Autodesk Inventor part; units mm, degrees
ref_plane "YZ Plane" through (0, 0, 0) normal (1, 0, 0) x (0, 1, 0)
ref_plane "XZ Plane" through (0, 0, 0) normal (0, 1, 0) x (-1, 0, 0)
ref_plane "XY Plane" through (0, 0, 0) normal (0, 0, 1) x (1, 0, 0)
sketch "Sketch1" plane through (0, 0, 0) normal (0, 1, 0) x (-1, 0, 0)
  line L0 (0, 0) -> (-36, 0)
  line L1 (-36, 0) -> (-36, -36)
  line L2 (-36, -36) -> (0, -36)
  line L3 (0, -36) -> (0, 0)
  circle A0 centre (-1.9445, -34.0555) radius 1.5
  circle A1 centre (-34.0555, -34.0555) radius 1.5
  circle A2 centre (-1.9445, -1.9445) radius 1.5
  circle A3 centre (-34.0555, -1.9445) radius 1.5
  line L4 (-6.1012, -34.6884) -> (-8.9666, -34.6884)
  line L5 (-8.9666, -34.6884) -> (-8.9666, -32.1278)
  line L6 (-8.9666, -32.1278) -> (-6.1012, -32.1278)
  line L7 (-6.1012, -32.1278) -> (-6.1012, -34.6884)
  line L8 (-11.5272, -34.6884) -> (-14.4536, -34.6884)
  line L9 (-14.4536, -34.6884) -> (-14.4536, -32.1278)
  line L10 (-14.4536, -32.1278) -> (-11.5272, -32.1278)
  line L11 (-11.5272, -32.1278) -> (-11.5272, -34.6884)
  line L12 (-17.5019, -34.6884) -> (-20.6111, -34.6884)
  line L13 (-20.6111, -34.6884) -> (-20.6111, -32.1278)
  line L14 (-20.6111, -32.1278) -> (-17.5019, -32.1278)
  line L15 (-17.5019, -32.1278) -> (-17.5019, -34.6884)
  line L16 (-23.9642, -34.6884) -> (-27.6831, -34.6884)
  line L17 (-27.6831, -34.6884) -> (-27.6831, -32.1278)
  line L18 (-27.6831, -32.1278) -> (-23.9642, -32.1278)
  line L19 (-23.9642, -32.1278) -> (-23.9642, -34.6884)
  line L20 (-34.6332, -30.055) -> (-31.9508, -30.055)
  line L21 (-31.9508, -30.055) -> (-31.9508, -27.5554)
  line L22 (-31.9508, -27.5554) -> (-34.6332, -27.5554)
  line L23 (-34.6332, -27.5554) -> (-34.6332, -30.055)
  line L24 (-34.6332, -24.0803) -> (-31.585, -24.0803)
  line L25 (-31.585, -24.0803) -> (-31.585, -21.9465)
  line L26 (-31.585, -21.9465) -> (-34.6332, -21.9465)
  line L27 (-34.6332, -21.9465) -> (-34.6332, -24.0803)
  line L28 (-34.6332, -18.8373) -> (-31.585, -18.8373)
  line L29 (-31.585, -18.8373) -> (-31.585, -16.2767)
  line L30 (-31.585, -16.2767) -> (-34.6332, -16.2767)
  line L31 (-34.6332, -16.2767) -> (-34.6332, -18.8373)
  line L32 (-34.0555, -11.8872) -> (-31.585, -11.8872)
  line L33 (-31.585, -11.8872) -> (-31.585, -7.6196)
  line L34 (-31.585, -7.6196) -> (-34.0555, -7.6196)
  line L35 (-34.0555, -7.6196) -> (-34.0555, -11.8872)
  line L36 (-28.7805, -2.6813) -> (-25.4884, -2.6813)
  line L37 (-25.4884, -2.6813) -> (-25.4884, -0.4445)
  line L38 (-25.4884, -0.4445) -> (-28.7805, -0.4445)
  line L39 (-28.7805, -0.4445) -> (-28.7805, -2.6813)
  line L40 (-21.0379, -2.6813) -> (-16.2825, -2.6813)
  line L41 (-16.2825, -2.6813) -> (-16.2825, -0.4445)
  line L42 (-16.2825, -0.4445) -> (-21.0379, -0.4445)
  line L43 (-21.0379, -0.4445) -> (-21.0379, -2.6813)
  line L44 (-13.661, -3.4445) -> (-10.4298, -3.4445)
  line L45 (-10.4298, -3.4445) -> (-10.4298, -1.0962)
  line L46 (-10.4298, -1.0962) -> (-13.661, -1.0962)
  line L47 (-13.661, -1.0962) -> (-13.661, -3.4445)
  line L48 (-6.1012, -3.4445) -> (-4.2113, -3.4445)
  line L49 (-4.2113, -3.4445) -> (-4.2113, -0.4445)
  line L50 (-4.2113, -0.4445) -> (-6.1012, -0.4445)
  line L51 (-6.1012, -0.4445) -> (-6.1012, -3.4445)
  line L52 (-2.4433, -7.6196) -> (-0.4445, -7.6196)
  line L53 (-0.4445, -7.6196) -> (-0.4445, -5.12)
  line L54 (-0.4445, -5.12) -> (-2.4433, -5.12)
  line L55 (-2.4433, -5.12) -> (-2.4433, -7.6196)
  line L56 (-2.4433, -13.5942) -> (-0.8582, -13.5942)
  line L57 (-0.8582, -13.5942) -> (-0.8582, -10.363)
  line L58 (-0.8582, -10.363) -> (-2.4433, -10.363)
  line L59 (-2.4433, -10.363) -> (-2.4433, -13.5942)
  line L60 (-3.4445, -19.6298) -> (-0.8582, -19.6298)
  line L61 (-0.8582, -19.6298) -> (-0.8582, -15.5451)
  line L62 (-0.8582, -15.5451) -> (-3.4445, -15.5451)
  line L63 (-3.4445, -15.5451) -> (-3.4445, -19.6298)
  line L64 (-2.931, -25.9703) -> (-0.8582, -25.9703)
  line L65 (-0.8582, -25.9703) -> (-0.8582, -22.6781)
  line L66 (-0.8582, -22.6781) -> (-2.931, -22.6781)
  line L67 (-2.931, -22.6781) -> (-2.931, -25.9703)
  line L68 (-2.931, -30.6646) -> (-0.8582, -30.6646)
  line L69 (-0.8582, -30.6646) -> (-0.8582, -28.8052)
  line L70 (-0.8582, -28.8052) -> (-2.931, -28.8052)
  line L71 (-2.931, -28.8052) -> (-2.931, -30.6646)
  line L72 (-27.6831, -30.055) -> (-6.528, -30.055)
  line L73 (-6.528, -30.055) -> (-6.528, -25.9703)
  line L74 (-6.528, -25.9703) -> (-27.6831, -25.9703)
  line L75 (-27.6831, -25.9703) -> (-27.6831, -30.055)
  line L76 (-6.528, -23.5926) -> (-27.6831, -23.5926)
  line L77 (-27.6831, -23.5926) -> (-27.6831, -18.8373)
  line L78 (-27.6831, -18.8373) -> (-6.528, -18.8373)
  line L79 (-6.528, -18.8373) -> (-6.528, -23.5926)
  line L80 (-25.8237, -9.2047) -> (-8.5399, -9.2047)
  line L81 (-8.5399, -9.2047) -> (-8.5399, -16.2767)
  line L82 (-8.5399, -16.2767) -> (-25.8237, -16.2767)
  line L83 (-25.8237, -16.2767) -> (-25.8237, -9.2047)
  dimension "d2" = 3
  dimension "d3" = 3
extrude "Extrusion1" add sketch "Sketch1" along normal blind 2 contours L3 L2 L1 L0 | L4 L5 L6 L7 | L8 L9 L10 L11 | L12 L13 L14 L15 | L16 L17 L18 L19 | L23 L22 L21 L20 | L27 L26 L25 L24 | L31 L30 L29 L28 | L35 L34 L33 L32 | L39 L38 L37 L36 | L43 L42 L41 L40 | L47 L46 L45 L44 | L51 L50 L49 L48 | L55 L54 L53 L52 | L59 L58 L57 L56 | L63 L62 L61 L60 | L67 L66 L65 L64 | L71 L70 L69 L68 | L75 L74 L73 L72 | L76 L77 L78 L79 | L80 L81 L82 L83
extrude "Extrusion2" add sketch "Sketch1" along normal blind 2.2 contours L4 L5 L6 L7 | L8 L9 L10 L11 | L12 L13 L14 L15 | L16 L17 L18 L19 | L23 L22 L21 L20 | L27 L26 L25 L24 | L31 L30 L29 L28 | L35 L34 L33 L32 | L39 L38 L37 L36 | L43 L42 L41 L40 | L47 L46 L45 L44 | L51 L50 L49 L48 | L55 L54 L53 L52 | L59 L58 L57 L56 | L63 L62 L61 L60 | L67 L66 L65 L64 | L71 L70 L69 L68 | L75 L74 L73 L72 | L76 L77 L78 L79 | L80 L81 L82 L83
properties part number "PDB 36x36"
Design review of the part built by this model. Coordinates are the model's own, in mm. Coordinates: 2 decimals unless noted, no trailing zeros. Loops run counter-clockwise (first coordinate to the right, second up) from the corner with the lowest first, then second, coordinate; pieces in that order, holes last.
Q1. The part is to be moulded in two halves that separate along X. For faces 1 (the face through (0, 1, -18)), 2 (the face through (34.251, 0.986, -35.543)), 3 (the face through (19, 2.2, -2)), say which applies: +X half, -X half, draft (parallel to the pull), parting line (faces both ways), or undercut.
Reported:
face 1: -X half
face 2: undercut
face 3: draft
Q2. We need section A-A on x = 2. State how many separate pieces and enclosed holes the cut face has, and give its area (3 significant figures).
Reported:
separate pieces: 3
enclosed holes: 0
area: 63.0 mm2
Q3. For pin 1 (12 mm diameter, centred on x = 10.5, z = -8, fed in from -Y), flat-tipped, find the tip position at first contact; note if it passes through.
Reported:
pin 1: stops at y = 0
Q4. We need section B-B on y = 1.2. State the section outline as (x, z) points.
Reported:
outline: (0, -36) - (36, -36) - (36, 0) - (0, 0) - close; hole circle Ø3 at (1.94, -34.06); hole circle Ø3 at (1.94, -1.94); hole circle Ø3 at (34.06, -34.06); hole circle Ø3 at (34.06, -1.94)
Q5. To check wall thickness, follow line 1 (Y direction, x = 17, z = -6); line 2 (Z direction, x = 3, y = 1.9); line 3 (X direction, y = 1.7, z = -33). State the ranges of each line that lie inside material, in increasing order.
Reported:
line 1: y = 0 to 2
line 2: z = -36 to -35.12, -32.99 to -3.01, -0.88 to 0
line 3: x = 0 to 0.88, 3.01 to 32.99, 35.12 to 36
